The listing builds one solid part. Answer for the finished solid, in the listing's coordinates (mm). Give positions to 0.01 mm unless a question says otherwise; leave off trailing zeros. Order: outer loops, then holes, each group sorted by start corner. A loop starts at its lowest first (then second) coordinate and runs counter-clockwise, first axis right, second up. Notation, with made-up numbers: (37, 55) - (41, 55) arc R36 cw to (41, 91) - close; hole circle Ø10 at (-5, 88.5). An arc over 180 degrees is marked (long way). Answer as CSV lines item,"result". Start each with the question number.
1. Section A-A on x = 61 is taken. Give the vertices of the cut face in (y, z).
2. Section D-D on x = -78.5 is taken. Give the vertices of the cut face in (y, z), and give its area (3 significant figures).
3. Consider line 1 along Y through (x, z) = (-43, 0.75); line 2 along Y through (x, z) = (-63, 2); line 3 along Y through (x, z) = (-29.5, 3.5). Determine where each line is inside the solid, lowest interval first. Write a range as [from, to].
4. Flat-ended cylindrical pins translate along their axes: pin 1 (2 mm diameter, centred on x = -50.5, z = 3, fed in from +Y); pin 2 (2 mm diameter, centred on x = 65.5, y = -29.5, fed in from +Z); pin 3 (0.6 mm diameter, centred on y = -48.5, z = 1.5, fed in from +X); pin 4 (2 mm diameter, centred on x = -71, y = -48.5, fed in from +Z). Find the tip coordinate at first contact, or state that the pin passes through.
5. Section B-B on y = -28.5 is taken. Give the vertices of the cut face in (x, z), and give its area (3 significant figures).
6. Section C-C on z = 3.35 is taken. Count the separate pieces of the cut face and the enclosed holes in it, and give its area (3 significant figures).
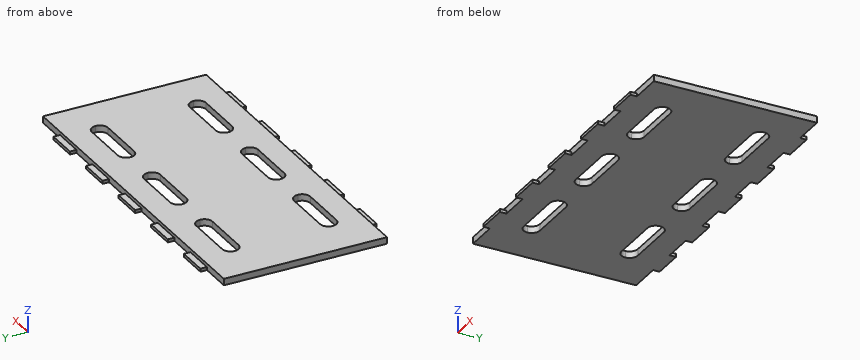
Autodesk Inventor part; units mm, degrees
ref_plane "YZ Plane" through (0, 0, 0) normal (1, 0, 0) x (0, 1, 0)
ref_plane "XZ Plane" through (0, 0, 0) normal (0, 1, 0) x (-1, 0, 0)
ref_plane "XY Plane" through (0, 0, 0) normal (0, 0, 1) x (1, 0, 0)
sketch "Sketch1" plane through (0, 0, 0) normal (0, 0, 1) x (1, 0, 0)
  line L0 (-100.0716, 53.5507) -> (107.9284, 53.5507)
  line L1 (107.9284, 53.5507) -> (107.9284, -46.4493)
  line L2 (107.9284, -46.4493) -> (-100.0716, -46.4493)
  line L3 (-100.0716, -46.4493) -> (-100.0716, 53.5507)
  point P0 (0, 0)
  dimension "d0" = 208
  dimension "d1" = 100
extrude "Extrusion1" add sketch "Sketch1" along normal blind 4
sketch "Sketch2" plane through (-100.0716, -46.4493, 0) normal (0, -1, 0) x (1, 0, 0)
  line L0 (0, 0) -> (208, 0)
  line L1 (19.5, 0) -> (38.5, 0)
  line L2 (38.5, 0) -> (38.5, 1.9)
  line L3 (38.5, 1.9) -> (19.5, 1.9)
  line L4 (19.5, 1.9) -> (19.5, 0)
  line L5 (0, 0) -> (0, 4)
  point P0 (100.0716, 0)
  point P1 (19.5, 0.95)
  dimension "d4" = 19
  dimension "d5" = 1.9
  dimension "d6" = 19.5
extrude "Extrusion2" add sketch "Sketch2" along normal blind 4
pattern_linear "Rectangular Pattern1" count 5 spacing 37.5 along (1, 0, 0) count 2 spacing 104 along (0, 1, 0) of "Extrusion2"
sketch "Sketch3" plane through (0, 0, 4) normal (0, 0, 1) x (1, 0, 0)
  line L0 (89.7284, -20.8493) -> (97.9284, -20.8493)
  line L1 (97.9284, -20.8493) -> (97.9284, -36.4493)
  line L2 (97.9284, -36.4493) -> (89.7284, -36.4493)
  line L3 (89.7284, -36.4493) -> (89.7284, -20.8493)
  line L4 (107.9284, 53.5507) -> (-100.0716, 53.5507)
  line L5 (-100.0716, 53.5507) -> (-100.0716, -46.4493)
  line L6 (107.9284, -46.4493) -> (107.9284, 53.5507)
  line L7 (-100.0716, -46.4493) -> (107.9284, -46.4493)
  point P0 (0, 0)
  dimension "d15" = 8.2
  dimension "d16" = 15.6
  dimension "d21" = 10
  dimension "d22" = 10
extrude "Extrusion3" [suppressed]
sketch "Sketch4" plane through (0, 0, 4) normal (0, 0, 1) x (1, 0, 0)
  line L0 (-75.0716, 38.5507) -> (-35.0716, 38.5507)
  line L1 (-35.0716, 38.5507) -> (-35.0716, 28.5507)
  line L2 (-35.0716, 28.5507) -> (-75.0716, 28.5507)
  line L3 (-75.0716, 28.5507) -> (-75.0716, 38.5507)
  line L4 (-15.0716, 38.5507) -> (24.9284, 38.5507)
  line L5 (24.9284, 38.5507) -> (24.9284, 28.5507)
  line L6 (24.9284, 28.5507) -> (-15.0716, 28.5507)
  line L7 (-15.0716, 28.5507) -> (-15.0716, 38.5507)
  line L8 (44.9284, 38.5507) -> (84.9284, 38.5507)
  line L9 (84.9284, 38.5507) -> (84.9284, 28.5507)
  line L10 (84.9284, 28.5507) -> (44.9284, 28.5507)
  line L11 (44.9284, 28.5507) -> (44.9284, 38.5507)
  line L12 (-100.0716, 53.5507) -> (-100.0716, -46.4493)
  line L13 (107.9284, 53.5507) -> (-100.0716, 53.5507)
  point P0 (0, 0)
  point P1 (-75.0716, 33.5507)
  point P2 (-15.0716, 33.5507)
  point P3 (-35.0716, 33.5507)
  point P4 (44.9284, 33.5507)
  point P5 (24.9284, 33.5507)
  dimension "d23" = 40
  dimension "d24" = 10
  dimension "d25" = 40
  dimension "d26" = 10
  dimension "d27" = 40
  dimension "d28" = 10
  dimension "d29" = 25
  dimension "d30" = 20
  dimension "d31" = 20
  dimension "d35" = 15
extrude "Extrusion4" cut sketch "Sketch4" against normal blind 10
fillet "Fillet1" radius 5 12 edges at (-75.0716, 38.5507, 2) (-75.0716, 28.5507, 2) (-35.0716, 28.5507, 2) (-35.0716, 38.5507, 2) (-15.0716, 38.5507, 2) (-15.0716, 28.5507, 2) (24.9284, 38.5507, 2) (24.9284, 28.5507, 2) (44.9284, 38.5507, 2) (44.9284, 28.5507, 2) (84.9284, 38.5507, 2) (84.9284, 28.5507, 2)
pattern_linear "Rectangular Pattern2" count 2 spacing 60 along (0, -1, 0) of "Extrusion4", "Fillet1"
properties part number "Enclosure_2"
Checks:
1,outline,"(-46.45, 0) - (-31.45, 0) - (-31.45, 4) - (-46.45, 4) - close; (-21.45, 0) - (28.55, 0) - (28.55, 4) - (-21.45, 4) - close; (38.55, 0) - (53.55, 0) - (53.55, 4) - (38.55, 4) - close"
2,outline,"(-50.45, 0) - (57.55, 0) - (57.55, 1.9) - (53.55, 1.9) - (53.55, 4) - (-46.45, 4) - (-46.45, 1.9) - (-50.45, 1.9) - close"
2,area,"415 mm²"
3,line 1,"y = [-50.45, -31.45], [-21.45, 28.55], [38.55, 57.55]"
3,line 2,"y = [-46.45, -31.45], [-21.45, 28.55], [38.55, 53.55]"
3,line 3,"y = [-46.45, 53.55]"
4,pin 1,"stops at y = 53.55"
4,pin 2,"passes through"
4,pin 3,"stops at x = 88.43"
4,pin 4,"stops at z = 1.9"
5,outline,"(-100.07, 0) - (-74.63, 0) - (-74.63, 4) - (-100.07, 4) - close; (-35.51, 0) - (-14.63, 0) - (-14.63, 4) - (-35.51, 4) - close; (24.49, 0) - (45.37, 0) - (45.37, 4) - (24.49, 4) - close; (84.49, 0) - (107.93, 0) - (107.93, 4) - (84.49, 4) - close"
5,area,"363 mm²"
6,separate pieces,"1"
6,enclosed holes,"6"
6,area,"18,500 mm²"
